Source: CAD feature listing. Evaluate the final solid. Frame: model axes, mm. A direction names the side the tool comes from. Round coordinates to 2 decimals unless told otherwise and drop trailing zeros. Write each loop counter-clockwise with the first axis right and the second up, starting at its lowest first coordinate (ties: lowest second). Pieces come first, ordered by that corner, then holes. Notation, with made-up numbers: M -27,70.25 L -13,70.25 A5 ccw -13,74.25 Z; hole C -19,-31.75 d7. An arc over 180 degrees is marked long. Use a Markdown table: item, result.
```python
from build123d import *

# Parameters (mm, degrees)
F0_R     = 45
F0_R_2   = 20.5
F1_DEPTH = 5
F0_R_3   = 17.5
F2_DEPTH = 2.5


# Not quite as in the source:
# - a fillet or chamfer that OpenCascade refuses, or shapes differently, is made with other operations: its cross-section is extruded or revolved along the edge and cut away or added


with BuildPart() as f1:
    # F0 (on Top) → F1 (new body)
    with BuildSketch(Plane.XY):
        Circle(F0_R)
        Circle(F0_R_2, mode=Mode.SUBTRACT)
    extrude(amount=F1_DEPTH)

    # F0 (on Top) → F2 (join)
    with BuildSketch(Plane.XY):
        Circle(F0_R_2)
        Circle(F0_R_3, mode=Mode.SUBTRACT)
    extrude(amount=F2_DEPTH)

    # F3: chamfer of 25 x 4.5 on 1 edges, made by hand

    # F3_s1 → F3_t2 (revolve, cut)
    with BuildSketch(Plane.XZ):
        Polygon((45, 0.5), (20, 5), (45, 5), align=None)
    revolve(axis=Axis((0, 0, 5), (0, 0, 1)), mode=Mode.SUBTRACT)


solid = f1.part
```
Q1. Line query: L1, parallel to Z at x = 10, y = -31; L2, parallel to Z at x = 29, y = 13.5; L3, parallel to X at y = 27.5, z = 0.3. Output: solid intervals per line, ascending.
Results are:
| item | result |
|---|---|
| L1 | 0 to 2.74 |
| L2 | 0 to 2.84 |
| L3 | -35.62 to 35.62 |
Q2. Reachability of faces 5 (the cylindrical face through (20.765, -39.923, 0.246)), 6 (the cylindrical face through (-4.444, -20.013, 3.688)) from +Z, -Z, +X, -X, +Y, -Y: full face, straight path, thin tool, end or side. Return the list, or none.
Results are:
| item | result |
|---|---|
| face 5 | +Z, -Z |
| face 6 | +Z |
Q3. Mould query, pull axis X, two halves, no side actions, for faces 1 (the flat face through (15.1, 9.2, 2.5)), 2 (the cylindrical face through (-13.887, -10.648, 1.232)), 3 (the conical face through (-17.212, -13.198, 4.696)), 4 (the flat face through (-1, -19, 0)). Classes: +X half, -X half, draft (parallel to the pull), parting line (faces both ways), or undercut.
Results are:
| item | result |
|---|---|
| face 1 | undercut |
| face 2 | undercut |
| face 3 | parting line |
| face 4 | draft |
Q4. First-contact query: pin 1 Ø4 at (x, y) = (-13, -35.5) entering from +Z (3 decimals); pin 2 Ø6 at (x, y) = (13, 22) entering from +Z. Flat tips, straight axial feed; report the tip coordinate or a pass-through.
Results are:
| item | result |
|---|---|
| pin 1 | z = 2.155 |
| pin 2 | z = 4.54 |
Q5. Section A-A on x = 0. Return loops of the section in (y, z).
Results are:
| item | result |
|---|---|
| outline | M -45,0 L -17.5,0 L -17.5,2.5 L -20.5,2.5 L -20.5,4.91 L -45,0.5 Z; M 17.5,0 L 45,0 L 45,0.5 L 20.5,4.91 L 20.5,2.5 L 17.5,2.5 Z |
